from build123d import *

# Parameters (mm, degrees)
SKETCH_2_R          = 1.5
CUT_EXTRUDE_1_DEPTH = 10
CHAMFER_1_SIZE      = 1


with BuildPart() as part:
    # 草圖1 → 旋轉1 (revolve)
    with BuildSketch(Plane(origin=(0, 0, 0), x_dir=(0, 0, -1), z_dir=(1, 0, 0)), mode=Mode.PRIVATE) as revolve_1_sk:
        with BuildLine():
            Line((2, 6), (58, 6))
            ThreePointArc((58, 6), (59.5, 4.5), (61, 6))
            Line((61, 6), (61, 8))
            Line((61, 8), (122, 8))
            Line((122, 8), (122, 5))
            ThreePointArc((122, 5), (123.5, 3.5), (125, 5))
            Line((125, 5), (142, 5))
            Line((142, 5), (142, 0))
            Line((142, 0), (0, 0))
            ThreePointArc((0, 0), (0.513167019, 3.16227766), (2, 6))
        make_face()
    revolve(revolve_1_sk.sketch.rotate(Axis((0, 0, 0), (0, 0, -1)), 90), axis=Axis((0, 0, 0), (0, 0, -1)))

    # 草圖2 → 除料-伸長1 (cut, symmetric)
    with BuildSketch(Plane(origin=(0, 0, 0), x_dir=(1, 0, 0), z_dir=(0, 1, 0))):
        with Locations(Location((0, 133, 0), (0, 0, 270))):
            Circle(SKETCH_2_R)
    extrude(amount=CUT_EXTRUDE_1_DEPTH, both=True, mode=Mode.SUBTRACT)

    # 導角1
    chamfer_1_edges = [part.edges().sort_by_distance(p)[0] for p in [
        (-5, 0, -142),
    ]]
    chamfer(chamfer_1_edges, length=CHAMFER_1_SIZE)


solid = part.part
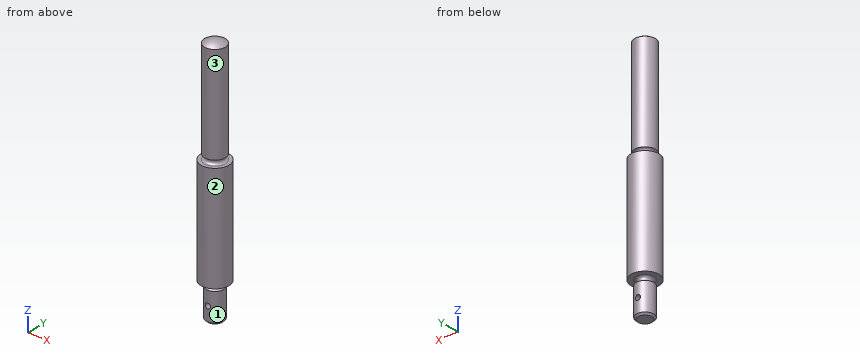
CAD build for the part. Positions are in the model's coordinates, mm. Face numbers are marked on the shaded views. A direction names the side the tool comes from. Give positions to 0.01 mm unless a question says otherwise; leave off trailing zeros. Loops run counter-clockwise (first coordinate to the right, second up) from the corner with the lowest first, then second, coordinate; pieces in that order, holes last. Notation, with made-up numbers: M 5,43.25 L 21,43.25 A29 cw 21,66.25 Z; hole C -9.5,1.25 d8. An arc over 180 degrees is marked long. Answer in a Markdown table with one row per item. Add a question column.
Item 1: Tool access for the marked faces 1, 2 and 3: list every direction of +Z, -Z, +X, -X, +Y, -Y with a clear straight run to the whole face (end or side of a thin tool).
Item 2: Probe probe 1 along Z at (x, y) = (-1, 4); probe 2 along Z at (x, y) = (4.25, -2.5); probe 3 along Y at (x, z) = (-0.5, -102). List the from-to ranges inside material, lowest first.
Item 3: Band-saw the part on B-B on y = 0. Give the cut face in (x, z), then the cut area to 3 significant figures.
Item 4: Band-saw the part on A-A on x = 0. Give the cut face in (y, z).
Item 5: Band-saw the part on C-C on z = -11. Give the cut face in (x, y), then the cut area to 3 significant figures.
Item 6: Drop flat-ended pins along their axis: P1, Ø5, axis at x = -3, z = -94.5, coming from the -Y side; P2, Ø1, axis at y = 4, z = -48.5, coming from the +X side; P3, Ø3, axis at x = -0.5, z = -35.5, coming from the -Y side. Give the stop position or say it passes through.
Item 7: Band-saw the part on D-D on z = -133. Give the cut face in (x, y), then the cut area to 3 significant figures.
Reply:
| question | item | result |
|---|---|---|
| 1 | face 1 | -Z |
| 1 | face 2 | +Z, -Z |
| 1 | face 3 | +Z |
| 2 | probe 1 | z = -141.88 to -134.12, -131.88 to -124.72, -122.28 to -0.89 |
| 2 | probe 2 | z = -141.07 to -125, -122 to -60.55, -58.45 to -1.3 |
| 2 | probe 3 | y = -7.98 to 7.98 |
| 3 | outline | M -8,-122 L -5,-122 A1.5 cw -5,-125 L -5,-141 L -4,-142 L 4,-142 L 5,-141 L 5,-125 A1.5 cw 5,-122 L 8,-122 L 8,-61 L 6,-61 A1.5 cw 6,-58 L 6,-2 A10 ccw -6,-2 L -6,-58 A1.5 cw -6,-61 L -8,-61 Z; hole C 0,-133 d3 |
| 3 | area | 1,880 mm^2 |
| 4 | outline | M -8,-122 L -5,-122 A1.5 cw -5,-125 L -5,-131.5 L 5,-131.5 L 5,-125 A1.5 cw 5,-122 L 8,-122 L 8,-61 L 6,-61 A1.5 cw 6,-58 L 6,-2 A10 ccw -6,-2 L -6,-58 A1.5 cw -6,-61 L -8,-61 Z; M -5,-141 L -4,-142 L 4,-142 L 5,-141 L 5,-134.5 L -5,-134.5 Z |
| 5 | outline | C 0,0 d12 |
| 5 | area | 113 mm^2 |
| 6 | P1 | stops at y = -7.98 |
| 6 | P2 | stops at x = 4.87 |
| 6 | P3 | stops at y = -6 |
| 7 | outline | M -1.5,-4.77 L -1.5,4.77 A5 ccw Z; M 1.5,-4.77 A5 ccw 1.5,4.77 Z |
| 7 | area | 49.0 mm^2 |
